```python
from build123d import *

# Parameters (mm, degrees)
SKETCH4_R           = 41.91
BOSS_EXTRUDE1_DEPTH = 6.35
SKETCH5_R           = 5
BOSS_EXTRUDE4_DEPTH = 27
BOSS_EXTRUDE5_START = 6.35
SKETCH7_R           = 41.91
BOSS_EXTRUDE5_DEPTH = 6.35


with BuildPart() as part:
    # Sketch4 → Boss-Extrude1 (new body)
    with BuildSketch(Plane(origin=(0, 0, 0), x_dir=(0, 0, -1), z_dir=(1, 0, 0))):
        Circle(SKETCH4_R)
    extrude(amount=BOSS_EXTRUDE1_DEPTH)

    # Sketch5 → Boss-Extrude4 (add)
    with BuildSketch(Plane.ZY):
        with Locations(Location((0, 0, 0), (0, 0, 180))):
            Circle(SKETCH5_R)
    extrude(amount=BOSS_EXTRUDE4_DEPTH)

    # Sketch7 → Boss-Extrude5 (add)
    with BuildSketch(Plane.ZY.offset(27).offset(BOSS_EXTRUDE5_START)):
        with Locations(Location((0, 0, 0), (0, 0, 180))):
            Circle(SKETCH7_R)
    extrude(amount=-BOSS_EXTRUDE5_DEPTH)


solid = part.part
```
Can you work these out from the model? Positions are in its coordinate system, mm. A direction names the side the tool comes from. Coordinates: 2 decimals unless noted, no trailing zeros. Loops run counter-clockwise (first coordinate to the right, second up) from the corner with the lowest first, then second, coordinate; pieces in that order, holes last. Notation, with made-up numbers: M 60.5,-38.75 L 96.5,-38.75 A21 cw 96.5,-22.75 Z; hole C -10,72 d1. An arc over 180 degrees is marked long. Put each result on its own line as item: value. Start each with the question number.
(1) Which directions (+Z, -Z, +X, -X, +Y, -Y) give clear straight access to the entire face, cutting with the end or side of a thin tool? Please do faces 1 (the face through (6.35, 1, 1)), 2 (the face through (-13, 0, 5)).
(2) Imagine slicing it at A-A on y = -25.5. List the corners of the cut face in (x, z) for me.
(3) Imagine slicing it at B-B on z = -10. List the corners of the cut face in (x, y) for me.
(4) Will these pins go through, and if not, where does the flat tip stop? pin 1 Ø3 at (x, y) = (-25, 31.5) entering from -Z; pin 2 Ø1 at (x, y) = (-22.5, 2) entering from +Z; pin 3 Ø5 at (x, y) = (0.5, 20) entering from -Z.
(5) I need wall thicknesses on probe 1 along X at (y, z) = (13, 27.5); probe 2 along Z at (x, y) = (-16.5, 0.5). Which ranges of each line are inside material? Lowest first, please.
(6) Imagine slicing it at C-C on z = 0. List the corners of the cut face in (x, y) for me, and give its area (3 significant figures).
Worked answers:
1. face 1: +Z, -Z, +X, +Y, -Y
1. face 2: none
2. outline: M -33.35,-33.26 L -27,-33.26 L -27,33.26 L -33.35,33.26 Z; M 0,-33.26 L 6.35,-33.26 L 6.35,33.26 L 0,33.26 Z
3. outline: M -33.35,-40.7 L -27,-40.7 L -27,40.7 L -33.35,40.7 Z; M 0,-40.7 L 6.35,-40.7 L 6.35,40.7 L 0,40.7 Z
4. pin 1: passes through
4. pin 2: stops at z = 4.77
4. pin 3: stops at z = -38.08
5. probe 1: x = -33.35 to -27, 0 to 6.35
5. probe 2: z = -4.97 to 4.97
6. outline: M -33.35,-41.91 L -27,-41.91 L -27,-5 L 0,-5 L 0,-41.91 L 6.35,-41.91 L 6.35,41.91 L 0,41.91 L 0,5 L -27,5 L -27,41.91 L -33.35,41.91 Z
6. area: 1,330 mm2
